```python
from build123d import *

# Parameters (mm, degrees)
F1_DEPTH = 2
F2_R     = 1


with BuildPart() as f1:
    # F0 (on Top) → F1 (new body, symmetric)
    with BuildSketch(Plane.XY):
        with BuildLine():
            ThreePointArc((9.5, 4.5), (9.2071067812, 5.2071067812), (8.5, 5.5))
            Line((8.5, 5.5), (-8.5, 5.5))
            ThreePointArc((-8.5, 5.5), (-9.2071067812, 5.2071067812), (-9.5, 4.5))
            Line((-9.5, 4.5), (-9.5, -4.5))
            ThreePointArc((-9.5, -4.5), (-9.2071067812, -5.2071067812), (-8.5, -5.5))
            Line((-8.5, -5.5), (8.5, -5.5))
            ThreePointArc((8.5, -5.5), (9.2071067812, -5.2071067812), (9.5, -4.5))
            Line((9.5, -4.5), (9.5, 4.5))
        make_face()
    extrude(amount=F1_DEPTH, both=True)

    # F2
    f2_edges = [f1.edges().sort_by_distance(p)[0] for p in [
        (0, -5.5, 2),
    ]]
    fillet(f2_edges, radius=F2_R)


solid = f1.part
```
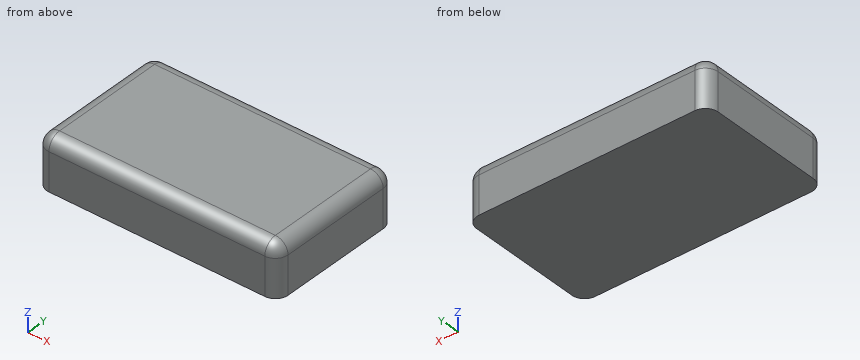
Verification items for the finished model (mm, model axes). Coordinates: 2 decimals unless noted, no trailing zeros. Loops run counter-clockwise (first coordinate to the right, second up) from the corner with the lowest first, then second, coordinate; pieces in that order, holes last. Notation, with made-up numbers: (79, -18.75) - (88, -18.75) arc R24 cw to (88, 2.25) - close; hole circle Ø8 at (8.25, -34). An arc over 180 degrees is marked (long way). Return JSON: item names as keys, results as strings.
1. Thickness scan on L1, parallel to Z at x = 8.75, y = 1; L2, parallel to X at y = 3, z = 1.6; L3, parallel to Y at x = 3.5, z = 1.3. Record the ranges inside material, lowest first.
Established:
{"L1": "z = -2 to 1.97", "L2": "x = -9.3 to 9.3", "L3": "y = -5.45 to 5.45"}
2. Section check A-A, the plane z = 1.7. Record the boundary of the cut face in (x, y).
Established:
{"outline": "(-9.21, -4.5) arc R0.71 ccw to (-8.5, -5.21) - (8.5, -5.21) arc R0.71 ccw to (9.21, -4.5) - (9.21, 4.5) arc R0.71 ccw to (8.5, 5.21) - (-8.5, 5.21) arc R0.71 ccw to (-9.21, 4.5) - close"}
3. Go/stop test with a flat-tipped pin: pin 1 (1.5 mm diameter, centred on x = 2.5, z = 1.5, fed in from -Y). Record where the tip stops, or that it passes through.
Established:
{"pin 1": "stops at y = -5.5"}
